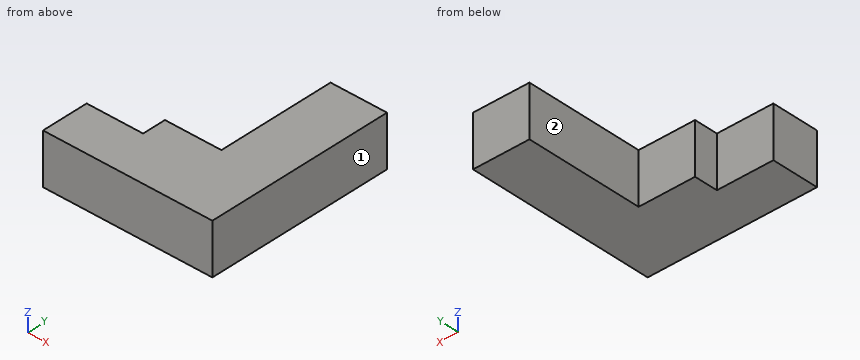
Autodesk Inventor part; units mm, degrees
ref_plane "YZ Plane" through (0, 0, 0) normal (1, 0, 0) x (0, 1, 0)
ref_plane "XZ Plane" through (0, 0, 0) normal (0, 1, 0) x (-1, 0, 0)
ref_plane "XY Plane" through (0, 0, 0) normal (0, 0, 1) x (1, 0, 0)
sketch "Sketch1" plane through (0, 0, 0) normal (0, 0, 1) x (1, 0, 0)
  line L0 (-900, -1000) -> (900, -1000)
  line L1 (900, -1000) -> (900, 1000)
  line L2 (900, 1000) -> (-900, 1000)
  line L3 (-900, 1000) -> (-900, -1000)
  line L4 (-900, -1000) -> (900, 1000) construction
  line L5 (900, -1000) -> (-900, 1000) construction
  point P0 (0, 0)
  dimension "d0" = 1000
  dimension "d1" = 900
extrude "Extrusion1" add sketch "Sketch1" against normal blind 540
sketch "Sketch2" plane through (0, 0, 0) normal (0, 0, 1) x (1, 0, 0)
  line L0 (-900, -1000) -> (900, -1000)
  line L1 (900, -1000) -> (900, 1000)
  line L2 (900, 1000) -> (-900, 1000)
  line L3 (-900, 1000) -> (-900, -1000)
  line L4 (900, -1000) -> (-900, -1000)
  line L5 (-900, -1000) -> (-900, -500)
  line L6 (-900, -1000) -> (-900, 1000)
  line L7 (-300, -500) -> (-300, -250)
  line L8 (-300, -250) -> (300, -250)
  line L9 (300, -250) -> (300, 1000)
  line L10 (-900, 1000) -> (-900, -500)
  line L11 (-300, -500) -> (-900, -500)
  point P0 (0, 0)
  point P1 (-300, -1000)
  point P2 (300, -1000)
  dimension "d4" = 600
  dimension "d5" = 600
  dimension "d6" = 600
  dimension "d7" = 500
  dimension "d8" = 1200
  dimension "d9" = 750
  dimension "d10" = 1500
extrude "Extrusion2" cut sketch "Sketch2" against normal up to next contours L3 L2 L9 L8 L7 L11
properties part number "data" material "ABS Plastic"
The model under review builds one solid part; all positions refer to its coordinate system, in mm. Face numbers are marked on the shaded views. A direction names the side the tool comes from. Give positions to 0.01 mm unless a question says otherwise; leave off trailing zeros. Write each loop counter-clockwise with the first axis right and the second up, starting at its lowest first coordinate (ties: lowest second). Pieces come first, ordered by that corner, then holes.
(1) Consider section B-B, the plane y = -200. Give the boundary of the cut face in (x, z), and give its area (3 significant figures).
(2) To check wall thickness, follow L1, parallel to X at y = 640, z = -226.5; L2, parallel to Y at x = -817.5, z = -43; L3, parallel to Y at x = -271, z = -28. State the ranges of each line that lie inside material, in increasing order.
(3) For P1, Ø5, axis at x = -331, z = -429, coming from the +Y side, flat-tipped, find the tip position at first contact; note if it passes through.
(4) Tool access review of the marked faces 1 and 2: name each direction out of +Z, -Z, +X, -X, +Y, -Y from which nothing blocks a thin tool from reaching the whole face with its end or side.
(5) Consider section C-C, the plane x = -429. Give the boundary of the cut face in (y, z), and give its area (3 significant figures).
(6) Consider section A-A, the plane z = -189. Give the boundary of the cut face in (x, y), and give its area (3 significant figures).
Returned:
1. outline: (300, -540) - (900, -540) - (900, 0) - (300, 0) - close
1. area: 324,000 mm2
2. L1: x = 300 to 900
2. L2: y = -1000 to -500
2. L3: y = -1000 to -250
3. P1: stops at y = -500
4. face 1: +Z, -Z, +X, +Y, -Y
4. face 2: +Z, -Z, -X, +Y
5. outline: (-1000, -540) - (-500, -540) - (-500, 0) - (-1000, 0) - close
5. area: 270,000 mm2
6. outline: (-900, -1000) - (900, -1000) - (900, 1000) - (300, 1000) - (300, -250) - (-300, -250) - (-300, -500) - (-900, -500) - close
6. area: 1,950,000 mm2
